Geometry: final body of the model. Coordinates: model frame, mm. Face numbers are marked on the shaded views. A direction names the side the tool comes from. Round coordinates to 2 decimals unless told otherwise and drop trailing zeros. Loops run counter-clockwise (first coordinate to the right, second up) from the corner with the lowest first, then second, coordinate; pieces in that order, holes last. Notation, with made-up numbers: (-13.75, 30.25) - (-6.75, 30.25) arc R26 ccw to (-6.75, 65.25) - close; hole circle Ø4 at (71.5, -0.5). An arc over 180 degrees is marked (long way). Answer as CSV lines item,"result".
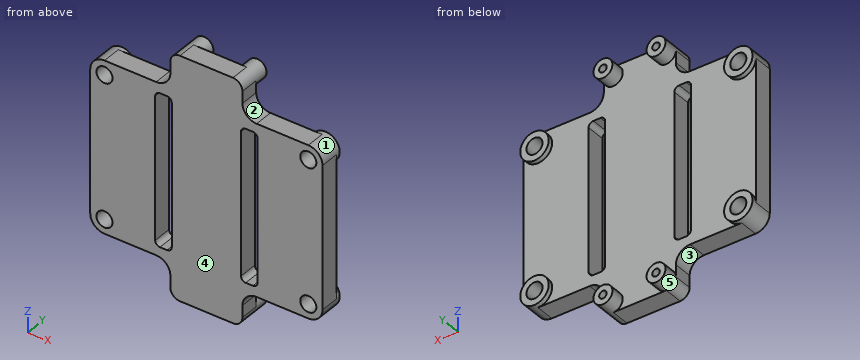
from build123d import *

# Parameters (mm, degrees)
SKETCH1_R               = 3
SKETCH1_R_2             = 1.7
BOSS_EXTRUDE1_DEPTH     = 5
BOSS_EXTRUDE1_2_DEPTH   = 5
BOSS_EXTRUDE1_3_DEPTH   = 5
BOSS_EXTRUDE1_4_DEPTH   = 5
BOSS_EXTRUDE2_DEPTH     = 4
CUT_EXTRUDE1_DEPTH      = 31.809901006
CUT_EXTRUDE1_DEPTH_BACK = 31.809901006
SKETCH1_2_R             = 1.7
SKETCH3_R               = 2
SKETCH3_R_2             = 0.8
BOSS_EXTRUDE3_DEPTH     = 7
BOSS_EXTRUDE3_2_DEPTH   = 7
BOSS_EXTRUDE3_3_DEPTH   = 7
BOSS_EXTRUDE3_4_DEPTH   = 7
BOSS_EXTRUDE4_DEPTH     = 4
CUT_EXTRUDE2_DEPTH      = 36.587919299
CUT_EXTRUDE2_DEPTH_BACK = 36.587919299
SKETCH6_W               = 3.5
SKETCH6_H               = 32
FILLET1_R               = 1
FILLET2_R               = 3


with BuildPart() as part:
    # Sketch1 → Boss-Extrude1 (new body)
    with BuildSketch(Plane(origin=(0, 0, 0), x_dir=(1, 0, 0), z_dir=(0, 1, 0))):
        with Locations(Location((-21.5, 15, 0), (0, 0, 270))):
            Circle(SKETCH1_R)
        with Locations(Location((-21.5, 15, 0), (0, 0, 270))):
            Circle(SKETCH1_R_2, mode=Mode.SUBTRACT)
    extrude(amount=BOSS_EXTRUDE1_DEPTH)



with BuildPart() as body_2:
    # Sketch1 → Boss-Extrude1 2 (new body)
    with BuildSketch(Plane(origin=(0, 0, 0), x_dir=(1, 0, 0), z_dir=(0, 1, 0))):
        with Locations(Location((-21.5, -15, 0), (0, 0, 270))):
            Circle(SKETCH1_R)
        with Locations(Location((-21.5, -15, 0), (0, 0, 270))):
            Circle(SKETCH1_R_2, mode=Mode.SUBTRACT)
    extrude(amount=BOSS_EXTRUDE1_2_DEPTH)


with BuildPart() as body_3:
    # Sketch1 → Boss-Extrude1 3 (new body)
    with BuildSketch(Plane(origin=(0, 0, 0), x_dir=(1, 0, 0), z_dir=(0, 1, 0))):
        with Locations(Location((21.5, -15, 0), (0, 0, 270))):
            Circle(SKETCH1_R)
        with Locations(Location((21.5, -15, 0), (0, 0, 270))):
            Circle(SKETCH1_R_2, mode=Mode.SUBTRACT)
    extrude(amount=BOSS_EXTRUDE1_3_DEPTH)


with BuildPart() as body_4:
    # Sketch1 → Boss-Extrude1 4 (new body)
    with BuildSketch(Plane(origin=(0, 0, 0), x_dir=(1, 0, 0), z_dir=(0, 1, 0))):
        with Locations(Location((21.5, 15, 0), (0, 0, 270))):
            Circle(SKETCH1_R)
        with Locations(Location((21.5, 15, 0), (0, 0, 270))):
            Circle(SKETCH1_R_2, mode=Mode.SUBTRACT)
    extrude(amount=BOSS_EXTRUDE1_4_DEPTH)


with BuildPart() as part_1:
    add(part.part)

    add(body_2.part)  # Boss-Extrude2 merges body 2

    add(body_3.part)  # Boss-Extrude2 merges body 3

    add(body_4.part)  # Boss-Extrude2 merges body 4
    # Sketch2 → Boss-Extrude2 (add)
    with BuildSketch(Plane(origin=(0, 0, 0), x_dir=(1, 0, 0), z_dir=(0, 1, 0))):
        with BuildLine():
            Line((-21.5, -18), (21.5, -18))
            ThreePointArc((21.5, -18), (23.621320344, -17.121320344), (24.5, -15))
            Line((24.5, -15), (24.5, 15))
            ThreePointArc((24.5, 15), (23.621320344, 17.121320344), (21.5, 18))
            Line((21.5, 18), (-21.5, 18))
            ThreePointArc((-21.5, 18), (-23.621320344, 17.121320344), (-24.5, 15))
            Line((-24.5, 15), (-24.5, -15))
            ThreePointArc((-24.5, -15), (-23.621320344, -17.121320344), (-21.5, -18))
        make_face()
    extrude(amount=BOSS_EXTRUDE2_DEPTH)

    # Sketch1<2> → Cut-Extrude1 (cut, two sides: drawn at the far end of the back side and taken through both)
    with BuildSketch(Plane(origin=(0, 0, 0), x_dir=(1, 0, 0), z_dir=(0, 1, 0)).offset(-CUT_EXTRUDE1_DEPTH_BACK)):
        with Locations(Location((-21.5, -15, 0), (0, 0, 270))):
            Circle(SKETCH1_2_R)
        with Locations(Location((-21.5, 15, 0), (0, 0, 270))):
            Circle(SKETCH1_2_R)
        with Locations(Location((21.5, 15, 0), (0, 0, 270))):
            Circle(SKETCH1_2_R)
        with Locations(Location((21.5, -15, 0), (0, 0, 270))):
            Circle(SKETCH1_2_R)
    extrude(amount=CUT_EXTRUDE1_DEPTH + CUT_EXTRUDE1_DEPTH_BACK, mode=Mode.SUBTRACT)



with BuildPart() as body_2_2:
    # Sketch3 → Boss-Extrude3 (new body)
    with BuildSketch(Plane(origin=(0, 0, 0), x_dir=(1, 0, 0), z_dir=(0, 1, 0))):
        with Locations(Location((-5.6, 23.5, 0), (0, 0, 270))):
            Circle(SKETCH3_R)
        with Locations(Location((-5.6, 23.5, 0), (0, 0, 270))):
            Circle(SKETCH3_R_2, mode=Mode.SUBTRACT)
    extrude(amount=BOSS_EXTRUDE3_DEPTH)


with BuildPart() as body_3_2:
    # Sketch3 → Boss-Extrude3 2 (new body)
    with BuildSketch(Plane(origin=(0, 0, 0), x_dir=(1, 0, 0), z_dir=(0, 1, 0))):
        with Locations(Location((5.6, 23.5, 0), (0, 0, 270))):
            Circle(SKETCH3_R)
        with Locations(Location((5.6, 23.5, 0), (0, 0, 270))):
            Circle(SKETCH3_R_2, mode=Mode.SUBTRACT)
    extrude(amount=BOSS_EXTRUDE3_2_DEPTH)


with BuildPart() as body_4_2:
    # Sketch3 → Boss-Extrude3 3 (new body)
    with BuildSketch(Plane(origin=(0, 0, 0), x_dir=(1, 0, 0), z_dir=(0, 1, 0))):
        with Locations(Location((-5.6, -23.5, 0), (0, 0, 270))):
            Circle(SKETCH3_R)
        with Locations(Location((-5.6, -23.5, 0), (0, 0, 270))):
            Circle(SKETCH3_R_2, mode=Mode.SUBTRACT)
    extrude(amount=BOSS_EXTRUDE3_3_DEPTH)


with BuildPart() as body_5:
    # Sketch3 → Boss-Extrude3 4 (new body)
    with BuildSketch(Plane(origin=(0, 0, 0), x_dir=(1, 0, 0), z_dir=(0, 1, 0))):
        with Locations(Location((5.6, -23.5, 0), (0, 0, 270))):
            Circle(SKETCH3_R)
        with Locations(Location((5.6, -23.5, 0), (0, 0, 270))):
            Circle(SKETCH3_R_2, mode=Mode.SUBTRACT)
    extrude(amount=BOSS_EXTRUDE3_4_DEPTH)


with BuildPart() as part_2:
    add(part_1.part)

    add(body_2_2.part)  # Boss-Extrude4 merges body 2 2

    add(body_3_2.part)  # Boss-Extrude4 merges body 3 2

    add(body_4_2.part)  # Boss-Extrude4 merges body 4 2

    add(body_5.part)  # Boss-Extrude4 merges body 5
    # Sketch4 → Boss-Extrude4 (add)
    with BuildSketch(Plane(origin=(0, 4, 0), x_dir=(1, 0, 0), z_dir=(0, 1, 0))):
        with BuildLine():
            Line((-5.6, -25.5), (5.6, -25.5))
            ThreePointArc((5.6, -25.5), (7.014213562, -24.914213562), (7.6, -23.5))
            Line((7.6, -23.5), (7.6, 23.5))
            ThreePointArc((7.6, 23.5), (7.014213562, 24.914213562), (5.6, 25.5))
            Line((5.6, 25.5), (-5.6, 25.5))
            ThreePointArc((-5.6, 25.5), (-7.014213562, 24.914213562), (-7.6, 23.5))
            Line((-7.6, 23.5), (-7.6, -23.5))
            ThreePointArc((-7.6, -23.5), (-7.014213562, -24.914213562), (-5.6, -25.5))
        make_face()
    extrude(amount=-BOSS_EXTRUDE4_DEPTH)

    # Sketch6 → Cut-Extrude2 (cut, two sides: drawn at the far end of the back side and taken through both)
    with BuildSketch(Plane(origin=(0, 4, 0), x_dir=(1, 0, 0), z_dir=(0, 1, 0)).offset(-CUT_EXTRUDE2_DEPTH_BACK)):
        with Locations((-9.05, 0)):
            Rectangle(SKETCH6_W, SKETCH6_H)
        with Locations((9.05, 0)):
            Rectangle(SKETCH6_W, SKETCH6_H)
    extrude(amount=CUT_EXTRUDE2_DEPTH + CUT_EXTRUDE2_DEPTH_BACK, mode=Mode.SUBTRACT)

    # Fillet1
    fillet1_edges = [part_2.edges().sort_by_distance(p)[0] for p in [
        (-10.8, 2, 16),
        (-10.8, 2, -16),
        (-7.3, 2, -16),
        (-7.3, 2, 16),
        (10.8, 2, -16),
        (10.8, 2, 16),
        (7.3, 2, 16),
        (7.3, 2, -16),
    ]]
    fillet(fillet1_edges, radius=FILLET1_R)

    # Fillet2
    fillet2_edges = [part_2.edges().sort_by_distance(p)[0] for p in [
        (-7.6, 2, 18),
        (-7.6, 2, -18),
        (7.6, 2, 18),
        (7.6, 2, -18),
    ]]
    fillet(fillet2_edges, radius=FILLET2_R)


solid = part_2.part
(1) Pin query (flat end, axial travel): P1, Ø0.5, axis at x = 5.5, z = -24, coming from the +Y side; P2, Ø1.8, axis at x = 21, z = -15.5, coming from the +Y side; P3, Ø1, axis at y = 1, z = -19, coming from the +X side; P4, Ø2, axis at y = 1, z = -22, coming from the +X side. Return the tip coordinate at first contact, or that it passes through.
Findings below:
P1,"y = 4"
P2,"through"
P3,"x = 8.94"
P4,"x = 7.6"
(2) Section D-D (y = 2.75). Give the number of separate pieces and of enclosed holes in the cut face, and give its area (3 significant figures).
Findings below:
separate pieces,"1"
enclosed holes,"6"
area,"1,730 mm2"
(3) Section A-A (y = 6.25). Output: boundary loops of the cut face in (x, z).
Findings below:
outline,"circle Ø4 at (-5.6, -23.5); circle Ø4 at (-5.6, 23.5); circle Ø4 at (5.6, -23.5); circle Ø4 at (5.6, 23.5); hole circle Ø1.6 at (-5.6, -23.5); hole circle Ø1.6 at (-5.6, 23.5); hole circle Ø1.6 at (5.6, -23.5); hole circle Ø1.6 at (5.6, 23.5)"
(4) Access query for the marked faces 1 and 2. Directions: +Z, -Z, +X, -X, +Y, -Y. A direction counts if a zero-diameter tool reaches every point of the face in a straight line with its end or side. Return the directions, or none.
Findings below:
face 1,"+Y"
face 2,"+Z, +X, +Y, -Y"
(5) Draft query along X for the marked faces 3, 4 and 5. Return one class per face: pulls with the +X half, pulls with the -X half, needs draft (parallel to the pull), parting line crosses it, or undercut.
Findings below:
face 3,"pulls with the -X half"
face 4,"needs draft"
face 5,"undercut"
(6) Section C-C (x = -16). Output: boundary loops of the cut face in (y, z), and give its area (3 significant figures).
Findings below:
outline,"(0, -18) - (4, -18) - (4, 18) - (0, 18) - close"
area,"144 mm2"
(7) Section B-B (z = 0). Output: boundary loops of the cut face in (x, y).
Findings below:
outline,"(-24.5, 0) - (-10.8, 0) - (-10.8, 4) - (-24.5, 4) - close; (-7.3, 0) - (7.3, 0) - (7.3, 4) - (-7.3, 4) - close; (10.8, 0) - (24.5, 0) - (24.5, 4) - (10.8, 4) - close"
(8) Material intervals for line 1 along Z through (x, y) = (-21.5, 3.4); line 2 along X through (y, z) = (3.75, 3.5); line 3 along X through (y, z) = (2.5, -15), sorted ascending.
Findings below:
line 1,"-18 to -16.7, -13.3 to 13.3, 16.7 to 18"
line 2,"-24.5 to -10.8, -7.3 to 7.3, 10.8 to 24.5"
line 3,"-24.5 to -23.2, -19.8 to -10.8, -7.3 to 7.3, 10.8 to 19.8, 23.2 to 24.5"
